```python
from build123d import *

# Parameters (mm, degrees)
BOSS_EXTRUDE1_DEPTH     = 398
CUT_EXTRUDE1_DEPTH      = 1867.759149714
CUT_EXTRUDE1_DEPTH_BACK = 1867.759149714
SKETCH3_R               = 3.96875
CUT_EXTRUDE3_DEPTH      = 1867.759149714


with BuildPart() as part:
    # Sketch1 → Boss-Extrude1 (new body)
    with BuildSketch(Plane.XY):
        Polygon((174.207835311, 1829.307995747), (105.642753947, 1532.32), (95.743154089, 1534.605502712), (164.308235453, 1831.593498459), align=None)
    extrude(amount=BOSS_EXTRUDE1_DEPTH)

    # Sketch2 → Cut-Extrude1 (cut, two sides: drawn at the far end of the back side and taken through both)
    with BuildSketch(Plane(origin=(-235.565521709, 54.384585889, 0), x_dir=(0, 0, -1), z_dir=(0.9743700647852336, -0.2249510543438718, 0)).offset(-CUT_EXTRUDE1_DEPTH_BACK)):
        with BuildLine():
            Line((-231.5, 1721.611186556), (-231.5, 1821.611186556))
            Line((-231.5, 1821.611186556), (-166.5, 1821.611186556))
            Line((-166.5, 1821.611186556), (-166.5, 1721.611186556))
            ThreePointArc((-166.5, 1721.611186556), (-199, 1689.111186556), (-231.5, 1721.611186556))
        make_face()
    extrude(amount=CUT_EXTRUDE1_DEPTH + CUT_EXTRUDE1_DEPTH_BACK, mode=Mode.SUBTRACT)

    # Sketch3 → Cut-Extrude3 (cut, through all)
    with BuildSketch(Plane(origin=(-235.565521709, 54.384585889, 0), x_dir=(0, 0, -1), z_dir=(0.9743700647852336, -0.2249510543438718, 0))):
        with Locations(Location((-389.5, 1669.211186556, 0), (0, 0, 90))):
            Circle(SKETCH3_R)
        with Locations(Location((-389.5, 1694.611186556, 0), (0, 0, 90))):
            Circle(SKETCH3_R)
        with Locations(Location((-389.5, 1720.011186556, 0), (0, 0, 90))):
            Circle(SKETCH3_R)
        with Locations(Location((-389.5, 1745.411186556, 0), (0, 0, 90))):
            Circle(SKETCH3_R)
        with Locations(Location((-389.5, 1770.811186556, 0), (0, 0, 90))):
            Circle(SKETCH3_R)
        with Locations(Location((-389.5, 1796.211186556, 0), (0, 0, 90))):
            Circle(SKETCH3_R)
        with Locations(Location((-389.5, 1542.211186556, 0), (0, 0, 90))):
            Circle(SKETCH3_R)
        with Locations(Location((-389.5, 1567.611186556, 0), (0, 0, 90))):
            Circle(SKETCH3_R)
        with Locations(Location((-389.5, 1593.011186556, 0), (0, 0, 90))):
            Circle(SKETCH3_R)
        with Locations(Location((-389.5, 1618.411186556, 0), (0, 0, 90))):
            Circle(SKETCH3_R)
        with Locations(Location((-389.5, 1643.811186556, 0), (0, 0, 90))):
            Circle(SKETCH3_R)
        with Locations(Location((-8.5, 1643.811186556, 0), (0, 0, 90))):
            Circle(SKETCH3_R)
        with Locations(Location((-8.5, 1618.411186556, 0), (0, 0, 90))):
            Circle(SKETCH3_R)
        with Locations(Location((-8.5, 1593.011186556, 0), (0, 0, 90))):
            Circle(SKETCH3_R)
        with Locations(Location((-8.5, 1567.611186556, 0), (0, 0, 90))):
            Circle(SKETCH3_R)
        with Locations(Location((-8.5, 1542.211186556, 0), (0, 0, 90))):
            Circle(SKETCH3_R)
        with Locations(Location((-8.5, 1796.211186556, 0), (0, 0, 90))):
            Circle(SKETCH3_R)
        with Locations(Location((-8.5, 1770.811186556, 0), (0, 0, 90))):
            Circle(SKETCH3_R)
        with Locations(Location((-8.5, 1745.411186556, 0), (0, 0, 90))):
            Circle(SKETCH3_R)
        with Locations(Location((-8.5, 1720.011186556, 0), (0, 0, 90))):
            Circle(SKETCH3_R)
        with Locations(Location((-8.5, 1694.611186556, 0), (0, 0, 90))):
            Circle(SKETCH3_R)
        with Locations(Location((-8.5, 1669.211186556, 0), (0, 0, 90))):
            Circle(SKETCH3_R)
    extrude(amount=-CUT_EXTRUDE3_DEPTH, mode=Mode.SUBTRACT)


solid = part.part
```
Work out the finished part from the listing and answer in its coordinate system (mm). Round coordinates to 2 decimals unless told otherwise and drop trailing zeros. Order: outer loops, then holes, each group sorted by start corner. A loop starts at its lowest first (then second) coordinate and runs counter-clockwise, first axis right, second up.
Q1. A cutting plane is placed at B-B, the plane y = 1694. Determine the outline of the cut face in (x, z), then the cut area to 3 significant figures.
Solution:
outline: (132.54, 0) - (142.97, 0) - (142.97, 398) - (132.54, 398) - close
area: 4,150 mm2
Q2. Find the intervals of material crossed by line 1 along Z through (x, y) = (148, 1741); line 2 along X through (y, z) = (1598, 89); line 3 along X through (y, z) = (1700, 146), in increasing order.
Solution:
line 1: z = 0 to 166.5, 231.5 to 398
line 2: x = 110.38 to 120.81
line 3: x = 133.93 to 144.35
Q3. The mould has two halves that part along Y. Classify faces 1 (the flat face through (140.405, 1682.893, 196.214)), 2 (the flat face through (158, 1781, 231.5)), 3 (the cylindrical face through (135.9, 1685.63, 9.69)): pulls with the +Y half, pulls with the -Y half, needs draft (parallel to the pull), parting line crosses it, or undercut.
Solution:
face 1: pulls with the -Y half
face 2: needs draft
face 3: undercut
Q4. Given pin 1 Ø3 at (y, z) = (1596.5, 84.5) entering from -X; pin 2 Ø8 at (y, z) = (1693, 119) entering from -X; pin 3 Ø10 at (x, y) = (125, 1705) entering from -Z, each flat-ended and moving along its own axis, determine where each tip first touches the part or whether it passes through.
Solution:
pin 1: stops at x = 109.69
pin 2: stops at x = 131.39
pin 3: passes through
Q5. A cutting plane is placed at A-A, the plane z = 136. Determine the outline of the cut face in (x, y), then the cut area to 3 significant figures.
Solution:
outline: (95.74, 1534.61) - (105.64, 1532.32) - (174.21, 1829.31) - (164.31, 1831.59) - close
area: 3,100 mm2
